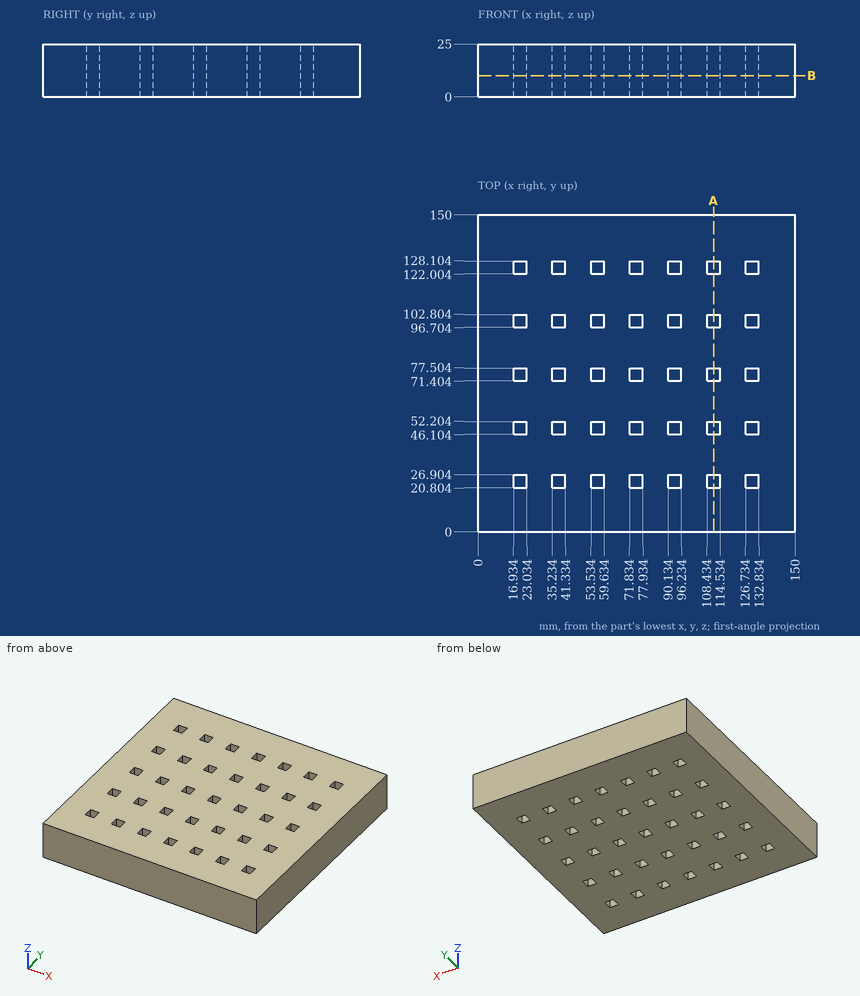
The drawing under review shows one solid part. Ordinate dimensions are in mm from its lowest x, y, z. Give positions to 0.01 mm unless a question says otherwise; leave off trailing zeros. Order: outer loops, then holes, each group sorted by start corner. A loop starts at its lowest first (then second) coordinate and runs counter-clockwise, first axis right, second up. Notation, with made-up numbers: M -32,48.5 L 4,48.5 A14 ccw 4,71.5 Z; hole C -8.5,81 d6. An arc over 180 degrees is marked long. Answer in a Markdown table with one row per item. Add a question column.
1. To check wall thickness, follow line 1 along Y through (x, z) = (58, 23.75). State the ranges of the line that lie inside material, in increasing order.
2. Add section B-B on z = 10. Count the separate pieces of the cut face and the enclosed holes in it, plus the area to 3 significant figures.
3. Add section A-A on x = 111.5. State the section outline as (y, z) points.
The answers:
| question | item | result |
|---|---|---|
| 1 | line 1 | 0 to 20.8, 26.9 to 46.1, 52.2 to 71.4, 77.5 to 96.7, 102.8 to 122, 128.1 to 150 |
| 2 | separate pieces | 1 |
| 2 | enclosed holes | 35 |
| 2 | area | 21,200 mm2 |
| 3 | outline | M 0,0 L 20.8,0 L 20.8,25 L 0,25 Z; M 26.9,0 L 46.1,0 L 46.1,25 L 26.9,25 Z; M 52.2,0 L 71.4,0 L 71.4,25 L 52.2,25 Z; M 77.5,0 L 96.7,0 L 96.7,25 L 77.5,25 Z; M 102.8,0 L 122,0 L 122,25 L 102.8,25 Z; M 128.1,0 L 150,0 L 150,25 L 128.1,25 Z |
